from build123d import *

# Parameters (mm, degrees)
F0_W      = 30
F0_H      = 20
F0_R      = 1.6
F1_DEPTH  = 5
F3_DEPTH  = 30
F7_DEPTH  = 7
F9_DEPTH  = 7
F10_SIZE  = 2.5
F11_R     = 5
F12_R     = 1.6200998357
F13_DEPTH = 30.001
F14_R     = 2
F17_DEPTH = 9


with BuildPart() as f1:
    # F0 (on Top) → F1 (new body)
    with BuildSketch(Plane.XY):
        Rectangle(F0_W, F0_H)
        with Locations((-8, 5.2767994255)):
            Circle(F0_R, mode=Mode.SUBTRACT)
        with Locations((0, 0.0767994255)):
            Circle(F0_R, mode=Mode.SUBTRACT)
        with Locations((8, 5.2767994255)):
            Circle(F0_R, mode=Mode.SUBTRACT)
    extrude(amount=F1_DEPTH)

    # F2 (on face) → F3 (join, through all)
    with BuildSketch(Plane(origin=(-15, 0, 0), x_dir=(0, -1, 0), z_dir=(-1, 0, 0))):
        with BuildLine():
            ThreePointArc((13.1, 5), (15.2920310217, 5.9079689783), (16.2, 8.1))
            ThreePointArc((16.2, 8.1), (13.1, 11.2), (10, 8.1))
            ThreePointArc((10, 8.1), (10.9079689783, 5.9079689783), (13.1, 5))
        make_face()
        with BuildLine():
            ThreePointArc((13.1, 5), (10.9079689783, 5.9079689783), (10, 8.1))
            ThreePointArc((10, 8.1), (8.1808280522, 5.8625059643), (5.4291286506, 5))
            Line((5.4291286506, 5), (10, 5))
            Line((10, 5), (10, 1.816622098))
            ThreePointArc((10, 1.816622098), (10.998268655, 3.9455916428), (13.1, 5))
        make_face()
    extrude(amount=-F3_DEPTH)

    # F6 (on offset) → F7 (cut)
    with BuildSketch(Plane.YZ.offset(11)):
        with BuildLine():
            ThreePointArc((-13.1, 5), (-10.9079689783, 5.9079689783), (-10, 8.1))
            ThreePointArc((-10, 8.1), (-15.2920310217, 10.2920310217), (-13.1, 5))
        make_face()
        with BuildLine():
            ThreePointArc((-5.4291286506, 5), (-8.1808280522, 5.8625059643), (-10, 8.1))
            ThreePointArc((-10, 8.1), (-10.9079689783, 5.9079689783), (-13.1, 5))
            ThreePointArc((-13.1, 5), (-10.998268655, 3.9455916428), (-10, 1.816622098))
            Line((-10, 1.816622098), (-10, 5))
            Line((-10, 5), (-5.4291286506, 5))
        make_face()
        with BuildLine():
            Line((-5.3136004135, 5), (-5.4291286506, 5))
            ThreePointArc((-5.4291286506, 5), (-5.371364532, 4.9996666743), (-5.3136004135, 5))
        make_face()
    extrude(amount=F7_DEPTH, mode=Mode.SUBTRACT)

    # F8 (on offset) → F9 (cut)
    with BuildSketch(Plane(origin=(-11, 0, 0), x_dir=(0, -1, 0), z_dir=(-1, 0, 0))):
        with BuildLine():
            ThreePointArc((13.1, 5), (15.2920310217, 5.9079689783), (16.2, 8.1))
            ThreePointArc((16.2, 8.1), (13.1, 11.2), (10, 8.1))
            ThreePointArc((10, 8.1), (10.9079689783, 5.9079689783), (13.1, 5))
        make_face()
        with BuildLine():
            ThreePointArc((5.3136004135, 5), (5.371364532, 4.9996666743), (5.4291286506, 5))
            Line((5.4291286506, 5), (5.3136004135, 5))
        make_face()
        with BuildLine():
            ThreePointArc((13.1, 5), (10.9079689783, 5.9079689783), (10, 8.1))
            ThreePointArc((10, 8.1), (8.1808280522, 5.8625059643), (5.4291286506, 5))
            Line((5.4291286506, 5), (10, 5))
            Line((10, 5), (10, 1.816622098))
            ThreePointArc((10, 1.816622098), (10.998268655, 3.9455916428), (13.1, 5))
        make_face()
    extrude(amount=F9_DEPTH, mode=Mode.SUBTRACT)

    # F10
    f10_edges = [f1.edges().sort_by_distance(p)[0] for p in [
        (-9.6, 5.276799, 5),
        (-1.6, 0.076799, 5),
        (6.4, 5.276799, 5),
    ]]
    chamfer(f10_edges, length=F10_SIZE)

    # F11
    f11_edges = [f1.edges().sort_by_distance(p)[0] for p in [
        (-15, 10, 2.5),
        (15, 10, 2.5),
    ]]
    fillet(f11_edges, radius=F11_R)

    # F12 (on face) → F13 (cut, through all)
    with BuildSketch(Plane(origin=(-15, 0, 0), x_dir=(0, -1, 0), z_dir=(-1, 0, 0))):
        with Locations((13.1, 8.1)):
            Circle(F12_R)
    extrude(amount=-F13_DEPTH, mode=Mode.SUBTRACT)

    # F14
    f14_edges = [f1.edges().sort_by_distance(p)[0] for p in [
        (-13, -10, 5),
        (13, -10, 5),
    ]]
    fillet(f14_edges, radius=F14_R)

    # F16 (on offset) → F17 (cut)
    with BuildSketch(Plane(origin=(-4.5, 0, 0), x_dir=(0, -1, 0), z_dir=(-1, 0, 0))):
        with BuildLine():
            ThreePointArc((10, 1.816622098), (10.998268655, 3.9455916428), (13.1, 5))
            ThreePointArc((13.1, 5), (15.2920310217, 10.2920310217), (10, 8.1))
            ThreePointArc((10, 8.1), (8.1808280522, 5.8625059643), (5.4291286506, 5))
            Line((5.4291286506, 5), (8, 5))
            ThreePointArc((8, 5), (9.4142135624, 4.4142135624), (10, 3))
            Line((10, 3), (10, 1.816622098))
        make_face()
    extrude(amount=-F17_DEPTH, mode=Mode.SUBTRACT)


solid = f1.part
The model under review builds one solid part; all positions refer to its coordinate system, in mm. A direction names the side the tool comes from. Round coordinates to 2 decimals unless told otherwise and drop trailing zeros. Write each loop counter-clockwise with the first axis right and the second up, starting at its lowest first coordinate (ties: lowest second). Pieces come first, ordered by that corner, then holes. Notation, with made-up numbers: M 32,-19 L 87,-19 A23 cw 87,11 Z; hole C 51,78 d2. An arc over 180 degrees is marked long. Answer as CSV lines item,"result". Start each with the question number.
Q1. Consider section A-A, the plane x = -8. Give the boundary of the cut face in (y, z), then the cut area to 3 significant figures.
Q2. Tool access review of faces 4 (the face through (0, -10, 1)), 5 (the face through (-0.06, -9.4, 4.43)), 6 (the face through (-1.366, -0.971, 2.621)): name each direction out of +Z, -Z, +X, -X, +Y, -Y from which nothing blocks a thin tool from reaching the whole face with its end or side.
Q3. Clearance check with flat-ended pins moving along their axes: P1, Ø5, axis at y = -13.1, z = 8.1, coming from the +X side; P2, Ø14.5, axis at x = -1, y = 0, coming from the +Z side; P3, Ø2, axis at x = 0.5, y = -8.5, coming from the +Z side. State where each tip first meets the part, or that it passes through.
Q4. Wall thickness on line 1 along Y through (x, z) = (0, 1.1); line 2 along X through (y, z) = (-9.5, 5); line 3 along Z through (x, y) = (-7.75, -13.1): over which ranges is each line inside the solid? List them lowest first.
Q5. Consider section C-C, the plane y = -13.5. Give the boundary of the cut face in (x, z).
Q6. The part is to be moulded in two halves that separate along X. For faces 1 (the face through (6.4, 5.3, 1.2)), 2 (the face through (-13, -7, 5)), 3 (the face through (-15, -2, 3)), say which applies: +X half, -X half, draft (parallel to the pull), parting line (faces both ways), or undercut.
Q7. Consider section D-D, the plane z = 1. Give the boundary of the cut face in (x, y), then the cut area to 3 significant figures.
Q8. Consider section B-B, the plane x = 0. Give the boundary of the cut face in (y, z).
Result set:
1,outline,"M -13.1,5 A3.59 cw -10,1.82 L -10,0 L 3.68,0 L 3.68,2.5 L 1.18,5 L -5.43,5 A5.01 cw -10,8.1 A3.1 ccw long Z; M 6.88,0 L 10,0 L 10,5 L 9.38,5 L 6.88,2.5 Z; hole C -13.1,8.1 d3.24"
1,area,"108 mm²"
2,face 4,"-Z, -Y"
2,face 5,"+Z, -Y"
2,face 6,"+Z"
3,P1,"stops at x = 11"
3,P2,"stops at z = 5.1"
3,P3,"stops at z = 5"
4,line 1,"y = -10 to -1.52, 1.68 to 10"
4,line 2,"x = -11 to -4.5, 4.5 to 11"
4,line 3,"z = 5 to 6.48, 9.72 to 11.2"
5,outline,"M -11,5.03 L -4.5,5.03 L -4.5,6.53 L -11,6.53 Z; M -11,9.67 L -4.5,9.67 L -4.5,11.17 L -11,11.17 Z; M 4.5,5.03 L 11,5.03 L 11,6.53 L 4.5,6.53 Z; M 4.5,9.67 L 11,9.67 L 11,11.17 L 4.5,11.17 Z"
6,face 1,"undercut"
6,face 2,"draft"
6,face 3,"-X half"
7,outline,"M -15,-10 L 15,-10 L 15,5 A5 ccw 10,10 L -10,10 A5 ccw -15,5 Z; hole C -8,5.28 d3.2; hole C 0,0.08 d3.2; hole C 8,5.28 d3.2"
7,area,"565 mm²"
8,outline,"M -10,0 L -1.52,0 L -1.52,2.5 L -4.02,5 L -8,5 A2 ccw -10,3 Z; M 1.68,0 L 10,0 L 10,5 L 4.18,5 L 1.68,2.5 Z"
